The listing builds one solid part. Answer for the finished solid, in the listing's coordinates (mm). A direction names the side the tool comes from. Coordinates: 2 decimals unless noted, no trailing zeros. Write each loop counter-clockwise with the first axis right and the second up, starting at its lowest first coordinate (ties: lowest second). Pieces come first, ordered by that corner, then holes.
from build123d import *

# Parameters (mm, degrees)
F0_W          = 182.1884661913
F0_H          = 90.4913619161
F1_DEPTH      = 25.4
F2_DEPTH      = 30.48
F4_DEPTH      = 12.7
F4_DEPTH_BACK = 101.6
F5_DEPTH      = 101.601
F6_R          = 9.1731778598
F7_DEPTH      = 55.881
F8_R          = 10.143728711
F9_DEPTH      = 55.881


with BuildPart() as f1:
    # F0 (on Top) → F1 (new body)
    with BuildSketch(Plane.XY):
        Rectangle(F0_W, F0_H)
    extrude(amount=F1_DEPTH)

    # F2 (add): a face of the model
    f2_faces = [f1.faces().sort_by_distance(p)[0] for p in [
        (0, 0, 25.4),
    ]]
    extrude(f2_faces, amount=F2_DEPTH)

    # F3 (on face) → F4 (join, two sides)
    with BuildSketch(Plane.XZ.offset(45.245680958)) as f4_sk:
        with BuildLine():
            ThreePointArc((36.8356928229, 55.88), (-1.8626e-06, 36.9552895427), (-36.8356965482, 55.88))
            Line((-36.8356965482, 55.88), (-48.5561415553, 55.88))
            ThreePointArc((-48.5561415553, 55.88), (1.3155639172, 26.427666579), (51.1872693896, 55.88))
            Line((51.1872693896, 55.88), (36.8356928229, 55.88))
        make_face()
    extrude(amount=F4_DEPTH)
    extrude(f4_sk.sketch, amount=-F4_DEPTH_BACK)

    # F5 (cut, through all): a face of the model
    f5_faces = [f1.faces().sort_by_distance(p)[0] for p in [
        (-1.8626e-06, -45.245680958, 48.1558042876),
    ]]
    extrude(f5_faces, amount=-F5_DEPTH, mode=Mode.SUBTRACT)

    # F6 (on face) → F7 (cut, through all)
    with BuildSketch(Plane.XY.offset(55.88)):
        with Locations((-72.8940144181, 0)):
            Circle(F6_R)
    extrude(amount=-F7_DEPTH, mode=Mode.SUBTRACT)

    # F8 (on face) → F9 (cut, through all)
    with BuildSketch(Plane.XY.offset(55.88)):
        with Locations((68.5885474086, 0)):
            Circle(F8_R)
    extrude(amount=-F9_DEPTH, mode=Mode.SUBTRACT)


solid = f1.part
Q1. Given pin 1 (5 mm diameter, centred on x = 54.5, z = 38, fed in from -Y); pin 2 (16 mm diameter, centred on x = 68.59, y = 0, fed in from +Z); pin 3 (8 mm diameter, centred on x = 43.5, z = 22.5, fed in from +Y); pin 4 (12 mm diameter, centred on x = -11.5, y = 20.5, fed in from +Z), each flat-ended and moving along its own axis, determine where each tip first touches the part or whether it passes through.
Answers below:
pin 1: stops at y = -45.25
pin 2: passes through
pin 3: stops at y = 45.25
pin 4: stops at z = 40.47
Q2. The part is cut by section B-B, the plane z = 44. Write down the section's boundary in (x, y).
Answers below:
outline: (-91.09, -45.25) - (-39.83, -45.25) - (-39.83, -57.95) - (-24.26, -57.95) - (-24.26, 56.35) - (-39.83, 56.35) - (-39.83, 45.25) - (-91.09, 45.25) - close; (24.26, -57.95) - (42.46, -57.95) - (42.46, -45.25) - (91.09, -45.25) - (91.09, 45.25) - (42.46, 45.25) - (42.46, 56.35) - (24.26, 56.35) - close; hole circle Ø18.35 at (-72.89, 0); hole circle Ø20.29 at (68.59, 0)
Q3. Which of the six approach directions +Z, -Z, +X, -X, +Y, -Y give full straight-line access (tool end or side, diameter ignored) to faces 1 (the face through (-1, 1, 0)), 2 (the face through (-1, 45.246, 21)), 3 (the face through (0.465, -51.507, 26.434))?
Answers below:
face 1: -Z, +X, -X, +Y, -Y
face 2: -Z, +Y
face 3: -Z, -Y
Q4. Determine the mould class of faces 4 (the face through (-1, -45.246, 21)), 5 (the face through (-91.094, -1, 28)), 6 (the face through (58.455, 0.446, 28.331)) for opening direction Y: released by +Y, released by -Y, zero draft, split by the parting line, or undercut.
Answers below:
face 4: released by -Y
face 5: zero draft
face 6: undercut
Q5. The part is cut by section A-A, the plane y = 0. Write down the section's boundary in (x, z), then the cut area to 4 significant figures.
Answers below:
outline: (-91.09, 0) - (-82.07, 0) - (-82.07, 55.88) - (-91.09, 55.88) - close; (-63.72, 0) - (58.44, 0) - (58.44, 55.88) - (36.84, 55.88) arc R45.31 cw to (-36.84, 55.88) - (-63.72, 55.88) - close; (78.73, 0) - (91.09, 0) - (91.09, 55.88) - (78.73, 55.88) - close
area: 7,045 mm2
Q6. The part is cut by section D-D, the plane x = 33. Write down the section's boundary in (y, z).
Answers below:
outline: (-57.95, 36.06) - (-45.25, 36.06) - (-45.25, 0) - (45.25, 0) - (45.25, 36.06) - (56.35, 36.06) - (56.35, 51.22) - (-57.95, 51.22) - close
Q7. Find the intervals of material crossed by probe 1 along X at (y, z) = (2.5, 48); probe 2 along Z at (x, y) = (-33, -38); probe 3 along Y at (x, z) = (42.5, 10), in increasing order.
Answers below:
probe 1: x = -91.09 to -81.72, -64.07 to -29.65, 29.65 to 58.76, 78.42 to 91.09
probe 2: z = 0 to 51.22
probe 3: y = -45.25 to 45.25
Q8. The part is cut by section C-C, the plane z = 34. Write down the section's boundary in (x, y).
Answers below:
outline: (-91.09, -45.25) - (-27.06, -45.25) - (-27.06, -57.95) - (29.69, -57.95) - (29.69, -45.25) - (91.09, -45.25) - (91.09, 45.25) - (29.69, 45.25) - (29.69, 56.35) - (-27.06, 56.35) - (-27.06, 45.25) - (-91.09, 45.25) - close; hole circle Ø18.35 at (-72.89, 0); hole circle Ø20.29 at (68.59, 0)
